```python
from build123d import *

# Parameters (mm, degrees)
SKETCH_2_R          = 1.6
EXTRUDE_1_DEPTH     = 4
EXTRUDE_1_2_DEPTH   = 4
SKETCH_3_W          = 7
SKETCH_3_H          = 4
EXTRUDE_2_DEPTH     = 30
SKETCH_4_W          = 47
SKETCH_4_H          = 8
EXTRUDE_3_DEPTH     = 4
SKETCH_5_R          = 1.1
CUT_EXTRUDE_1_DEPTH = 42.893116752


with BuildPart() as part:
    # Sketch 2 → Extrude 1 (new body)
    with BuildSketch(Plane(origin=(0, 0, 0), x_dir=(1, 0, 0), z_dir=(0, 1, 0))):
        Polygon((-23.5, 3.41991342), (-16.5, 3.41991342), (-16.5, -3.41991342), (-16.5, -7.41991342), (-23.5, -7.41991342), (-23.5, -3.41991342), align=None)
        with Locations(Location((-20, 0, 0), (0, 0, 270))):
            Circle(SKETCH_2_R, mode=Mode.SUBTRACT)
    extrude(amount=EXTRUDE_1_DEPTH)



with BuildPart() as body_2:
    # Sketch 2 → Extrude 1 2 (new body)
    with BuildSketch(Plane(origin=(0, 0, 0), x_dir=(1, 0, 0), z_dir=(0, 1, 0))):
        Polygon((23.5, -7.41991342), (23.5, -3.41991342), (23.5, 3.41991342), (16.5, 3.41991342), (16.5, -3.41991342), (16.5, -7.41991342), align=None)
        with Locations(Location((20, 0, 0), (0, 0, 90))):
            Circle(SKETCH_2_R, mode=Mode.SUBTRACT)
    extrude(amount=EXTRUDE_1_2_DEPTH)


with BuildPart() as part_1:
    add(part.part)

    add(body_2.part)  # Extrude 2 merges body 2
    # Sketch 3 → Extrude 2 (add)
    with BuildSketch(Plane(origin=(0, 4, 0), x_dir=(1, 0, 0), z_dir=(0, 1, 0))):
        with Locations((-20, -5.41991342)):
            Rectangle(SKETCH_3_W, SKETCH_3_H)
        with Locations((20, -5.41991342)):
            Rectangle(SKETCH_3_W, SKETCH_3_H)
    extrude(amount=EXTRUDE_2_DEPTH)

    # Sketch 4 → Extrude 3 (add)
    with BuildSketch(Plane(origin=(0, 0, 3.41991342), x_dir=(-1, 0, 0), z_dir=(0, 0, -1))):
        with Locations((0, 30)):
            Rectangle(SKETCH_4_W, SKETCH_4_H)
    extrude(amount=-EXTRUDE_3_DEPTH)

    # Sketch 5 → Cut-Extrude 1 (cut, through all)
    with BuildSketch(Plane(origin=(0, 0, 3.41991342), x_dir=(-1, 0, 0), z_dir=(0, 0, -1))):
        with Locations((-3.25, 31.1)):
            Circle(SKETCH_5_R)
        with Locations(Location((3.25, 31.1, 0), (0, 0, 180))):
            Circle(SKETCH_5_R)
    extrude(amount=-CUT_EXTRUDE_1_DEPTH, mode=Mode.SUBTRACT)


solid = part_1.part
```
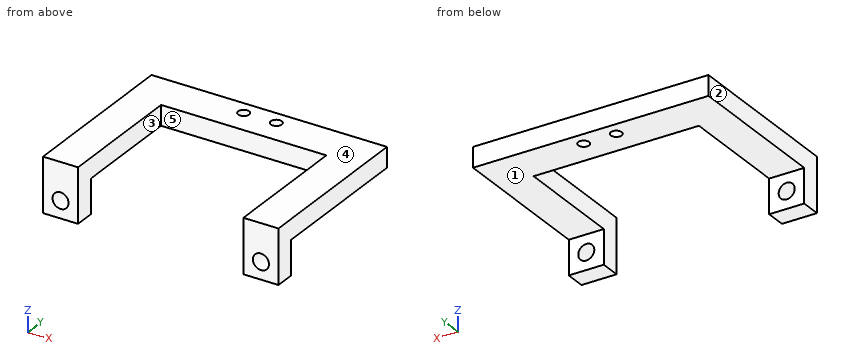
Design review of the part built by this model. Coordinates are the model's own, in mm. Face numbers are marked on the shaded views. A direction names the side the tool comes from. Coordinates: 2 decimals unless noted, no trailing zeros. Loops run counter-clockwise (first coordinate to the right, second up) from the corner with the lowest first, then second, coordinate; pieces in that order, holes last.
Q1. To check wall thickness, follow line 1 (X direction, y = 23.5, z = 6.5); line 2 (X direction, y = 3, z = 0); line 3 (Y direction, x = 3.25, z = 5.65). State the ranges of each line that lie inside material, in increasing order.
Reported:
line 1: x = -23.5 to -16.5, 16.5 to 23.5
line 2: x = -23.5 to -21.6, -18.4 to -16.5, 16.5 to 18.4, 21.6 to 23.5
line 3: y = 26 to 30, 32.2 to 34
Q2. We need section C-C on y = 7. State the section outline as (x, z) points, and give its area (3 significant figures).
Reported:
outline: (-23.5, 3.42) - (-16.5, 3.42) - (-16.5, 7.42) - (-23.5, 7.42) - close; (16.5, 3.42) - (23.5, 3.42) - (23.5, 7.42) - (16.5, 7.42) - close
area: 56.0 mm2
Q3. For pin 1 (4 mm diameter, centred on x = 20, z = 0, fed in from +Y); pin 2 (10 mm diameter, centred on x = 6.5, y = 27, fed in from -Z); pin 3 (4.5 mm diameter, centred on x = -3.5, z = 4.5, fed in from -Y), all flat-tipped, find the tip position at first contact; note any pin that passes through.
Reported:
pin 1: stops at y = 4
pin 2: stops at z = 3.42
pin 3: stops at y = 26
Q4. The part is to be moulded in two halves that separate along X. For the marked faces 1, 2 and 3, say which applies: +X half, -X half, draft (parallel to the pull), parting line (faces both ways), or undercut.
Reported:
face 1: draft
face 2: -X half
face 3: undercut
Q5. Tool access review of the marked faces 4 and 5: name each direction out of +Z, -Z, +X, -X, +Y, -Y from which nothing blocks a thin tool from reaching the whole face with its end or side.
Reported:
face 4: +Z, +X, -X, +Y, -Y
face 5: +Z, -Z, -Y
Q6. We need section A-A on y = 31.1. State the section outline as (x, z) points, and give its area (3 significant figures).
Reported:
outline: (-23.5, 3.42) - (-4.35, 3.42) - (-4.35, 7.42) - (-23.5, 7.42) - close; (-2.15, 3.42) - (2.15, 3.42) - (2.15, 7.42) - (-2.15, 7.42) - close; (4.35, 3.42) - (23.5, 3.42) - (23.5, 7.42) - (4.35, 7.42) - close
area: 170 mm2
Q7. We need section D-D on z = 5.5. State the section outline as (x, y) points.
Reported:
outline: (-23.5, 0) - (-16.5, 0) - (-16.5, 26) - (16.5, 26) - (16.5, 0) - (23.5, 0) - (23.5, 34) - (-23.5, 34) - close; hole circle Ø2.2 at (-3.25, 31.1); hole circle Ø2.2 at (3.25, 31.1)
Q8. We need section B-B on x = -3.25. State the section outline as (y, z) points.
Reported:
outline: (26, 3.42) - (30, 3.42) - (30, 7.42) - (26, 7.42) - close; (32.2, 3.42) - (34, 3.42) - (34, 7.42) - (32.2, 7.42) - close
